Here's how the part is built. I have some questions about the finished solid (model axes, mm). Give positions to 0.01 mm unless a question says otherwise; leave off trailing zeros. Loops run counter-clockwise (first coordinate to the right, second up) from the corner with the lowest first, then second, coordinate; pieces in that order, holes last. Notation, with made-up numbers: (66.5, -0.75) - (91.5, -0.75) arc R29 cw to (91.5, 19.25) - close; hole circle Ø11 at (-21.75, 42.5). An arc over 180 degrees is marked (long way). Use one line per item in the form item = value.
from build123d import *

# Parameters (mm, degrees)
SKETCH_1_W = 10
SKETCH_1_H = 200
FILLET_2_R = 10


with BuildPart() as part:
    # Эскиз1 → Повернуть1 (revolve)
    with BuildSketch(Plane.XY, mode=Mode.PRIVATE) as revolve_1_sk:
        with Locations((50, 0)):
            Rectangle(SKETCH_1_W, SKETCH_1_H)
    revolve(revolve_1_sk.sketch.rotate(Axis((0, -110.603092707, 0), (0, 1, 0)), 90), axis=Axis((0, -110.603092707, 0), (0, 1, 0)))

    # Скругление2
    fillet_2_edges = [part.edges().sort_by_distance(p)[0] for p in [
        (0, 100, 45),
    ]]
    fillet(fillet_2_edges, radius=FILLET_2_R - 0.0001)  # a hair under: the kernel refuses the full size


solid = part.part
(1) For P1, Ø10, axis at y = -44, z = 42, coming from the +X side; P2, Ø6, axis at y = 11, z = -14.5, coming from the -X side; P3, Ø10, axis at y = -33.5, z = 25, coming from the -X side, each with a flat end and sliding along its axis, tell me the tip position at first contact or that it passes through.
Geometry says:
P1 = 40.69
P2 = -53.78
P3 = -51.23
(2) If I drill on probe 1 along X at (y, z) = (-53, 0); probe 2 along X at (y, z) = (-33.5, -11); probe 3 along Z at (x, y) = (5.5, -56), over which ranges is the centre line in solid material (lowest first)?
Geometry says:
probe_1 = -55 to -45, 45 to 55
probe_2 = -53.89 to -43.63, 43.63 to 53.89
probe_3 = -54.72 to -44.66, 44.66 to 54.72
(3) Thinking about a two-plate mould opening in X: for faces 1 (the flat face through (40, -100, -21)), 2 (the cylindrical face through (39.923, -3.67, -20.765)), 3 (the cylindrical face through (48.794, 1.4, -25.379)), which applies, pulls with the +X half, pulls with the -X half, needs draft (parallel to the pull), parting line crosses it, or undercut?
Geometry says:
face_1 = needs draft
face_2 = undercut
face_3 = parting line crosses it
(4) If we section it at C-C (y = 77.5): List the corners of the cut face in (x, z) for me.
Geometry says:
outline = circle Ø110 at (0, 0); hole circle Ø90 at (0, 0)
